The model under review builds one solid part; all positions refer to its coordinate system, in mm. A direction names the side the tool comes from. Give positions to 0.01 mm unless a question says otherwise; leave off trailing zeros. Order: outer loops, then holes, each group sorted by start corner. A loop starts at its lowest first (then second) coordinate and runs counter-clockwise, first axis right, second up. Notation, with made-up numbers: (70, 73) - (125, 73) arc R17 cw to (125, 84) - close; hole circle Ø5 at (69.5, 81). An arc over 180 degrees is marked (long way). Use CSV: the item, a comma, the result in double quotes.
```python
from build123d import *

# Parameters (mm, degrees)
MASTER_SKETCH_R       = 52.451
MASTER_SKETCH_R_2     = 9.525
MASTER_SKETCH_R_3     = 27.4955
MASTER_SKETCH_R_4     = 6.5
BOSS_EXTRUDE2_DEPTH   = 4.7625
F_5_0MM_DOWEL_HOLE1_D = 5
CIRPATTERN4_COUNT     = 4
M6_CLEARANCE_HOLE4_D  = 6.6
M8_CLEARANCE_HOLE1_D  = 9
CIRPATTERN3_COUNT     = 9
CUT_EXTRUDE2_DEPTH    = 281.006585399
CUT_EXTRUDE3_DEPTH    = 281.006585399
FILLET1_R             = 2.54


with BuildPart() as part:
    # Master Sketch → Boss-Extrude2 (new, symmetric)
    # profile 1 of 5: a face of its own
    with BuildSketch(Plane(origin=(0, 0, 0), x_dir=(1, 0, 0), z_dir=(0, 1, 0))):
        with BuildLine():
            ThreePointArc((-8.636, 127), (-36.396097826, 84.787887478), (-86.152093601, 93.552952189))
            Line((-86.152093601, 93.552952189), (-6.534964144, 18.470363023))
            ThreePointArc((-6.534964144, 18.470363023), (-3.773598517, 34.145603423), (9.525, 25.4))
            ThreePointArc((9.525, 25.4), (8.799952547, 21.754940307), (6.735192091, 18.664807909))
            Line((6.735192091, 18.664807909), (23.243231805, 35.172847623))
            ThreePointArc((23.243231805, 35.172847623), (46.587798651, 48.47044475), (73.449951392, 48.001786374))
            Line((73.449951392, 48.001786374), (207.780426054, 8.637567885))
            ThreePointArc((207.780426054, 8.637567885), (203.365353978, 24.134749361), (219.252182081, 21.439533608))
            Line((219.252182081, 21.439533608), (190.024652545, 91.633132973))
            ThreePointArc((190.024652545, 91.633132973), (188.9083984, 102.577169262), (194.028954622, 112.313588397))
            Line((194.028954622, 112.313588397), (211.918529766, 130.503579499))
            ThreePointArc((211.918529766, 130.503579499), (196.325302338, 133.542806943), (205.218502749, 146.70702479))
            Line((205.218502749, 146.70702479), (174.268477279, 147.002761769))
            ThreePointArc((174.268477279, 147.002761769), (167.967389572, 148.13899706), (162.39865644, 151.298735696))
            ThreePointArc((162.39865644, 151.298735696), (144.003054669, 161.678519087), (123.19, 165.2778))
            Line((123.19, 165.2778), (-50.637408401, 172.802043535))
            ThreePointArc((-50.637408401, 172.802043535), (-20.726046555, 158.072276629), (-8.636, 127))
        make_face()
        with Locations(Location((123.19, 103.3018, 0), (0, 0, 90))):
            Circle(MASTER_SKETCH_R, mode=Mode.SUBTRACT)
    # profile 2 of 5: a face of its own
    with BuildSketch(Plane(origin=(0, 0, 0), x_dir=(1, 0, 0), z_dir=(0, 1, 0))):
        with Locations((210.458993886, 17.778185992)):
            Circle(MASTER_SKETCH_R_2)
    # profile 3 of 5: a face of its own
    with BuildSketch(Plane(origin=(0, 0, 0), x_dir=(1, 0, 0), z_dir=(0, 1, 0))):
        with Locations((0, 25.4)):
            Circle(MASTER_SKETCH_R_2)
    # profile 4 of 5: a face of its own
    with BuildSketch(Plane(origin=(0, 0, 0), x_dir=(1, 0, 0), z_dir=(0, 1, 0))):
        with Locations((205.12749261, 137.182459595)):
            Circle(MASTER_SKETCH_R_2)
    # profile 5 of 5: a face of its own
    with BuildSketch(Plane(origin=(0, 0, 0), x_dir=(1, 0, 0), z_dir=(0, 1, 0))):
        with BuildLine():
            ThreePointArc((-54.61, 172.974), (-97.337644752, 143.969297274), (-86.152093601, 93.552952189))
            ThreePointArc((-86.152093601, 93.552952189), (-36.396097826, 84.787887478), (-8.636, 127))
            ThreePointArc((-8.636, 127), (-20.726046555, 158.072276629), (-50.637408401, 172.802043535))
            Line((-50.637408401, 172.802043535), (-54.61, 172.974))
        make_face()
        with Locations(Location((-54.61, 127, 0), (0, 0, 90))):
            Circle(MASTER_SKETCH_R_3, mode=Mode.SUBTRACT)
        with Locations(Location((-67.94878559, 163.648012211, 0), (0, 0, 90))):
            Circle(MASTER_SKETCH_R_4, mode=Mode.SUBTRACT)
        with Locations(Location((-41.27121441, 163.648012211, 0), (0, 0, 90))):
            Circle(MASTER_SKETCH_R_4, mode=Mode.SUBTRACT)
    extrude(amount=BOSS_EXTRUDE2_DEPTH, both=True)

    # Ø5.0mm Dowel Hole1 (through all)
    with Locations(Plane(origin=(0, 4.7625, 0), x_dir=(1, 0, 0), z_dir=(0, 1, 0))):
        with Locations((123.19, 160.4518)):
            f_5_0mm_dowel_hole1 = Hole(F_5_0MM_DOWEL_HOLE1_D / 2)

    # CirPattern4: Ø5.0mm Dowel Hole1 ×4 about axis
    cirpattern4_axis = Axis((123.19, 0, -103.3018), (0, 1, 0))
    for i in range(1, CIRPATTERN4_COUNT):
        add(f_5_0mm_dowel_hole1.rotate(cirpattern4_axis, i * 360 / CIRPATTERN4_COUNT), mode=Mode.SUBTRACT)

    # M6 Clearance Hole4 (through all)
    with Locations(Plane(origin=(0, 4.7625, 0), x_dir=(1, 0, 0), z_dir=(0, 1, 0))):
        with Locations((205.12749261, 137.182459595), (210.458993886, 17.778185992), (0, 25.4)):
            Hole(M6_CLEARANCE_HOLE4_D / 2)

    # M8 Clearance Hole1 (through all)
    with Locations(Plane(origin=(0, 4.7625, 0), x_dir=(1, 0, 0), z_dir=(0, 1, 0))):
        with Locations((-54.61, 166)):
            m8_clearance_hole1 = Hole(M8_CLEARANCE_HOLE1_D / 2)

    # CirPattern3: M8 Clearance Hole1 ×9 about axis
    cirpattern3_axis = Axis((-54.61, 0, -127), (0, 1, 0))
    for i in range(1, CIRPATTERN3_COUNT):
        add(m8_clearance_hole1.rotate(cirpattern3_axis, i * 360 / CIRPATTERN3_COUNT), mode=Mode.SUBTRACT)

    # Topology 3 → Cut-Extrude2 (cut, through all)
    with BuildSketch(Plane(origin=(0, 4.7625, 0), x_dir=(1, 0, 0), z_dir=(0, 1, 0))):
        with BuildLine():
            ThreePointArc((17.44176984, 42.84176984), (-0.146601343, 35.405008389), (-17.945313453, 42.323250142))
            Line((-17.945313453, 42.323250142), (-33.032755262, 56.551396808))
            ThreePointArc((-33.032755262, 56.551396808), (-37.018106584, 65.604842248), (-33.299725858, 74.771168898))
            Line((-33.299725858, 74.771168898), (-25.157987823, 82.912906934))
            ThreePointArc((-25.157987823, 82.912906934), (-16.98904431, 89.126755018), (-7.457826773, 92.934567826))
            Line((-7.457826773, 92.934567826), (46.455825782, 106.412980965))
            ThreePointArc((46.455825782, 106.412980965), (54.31445648, 104.914466858), (58.258837609, 97.954188236))
            ThreePointArc((58.258837609, 97.954188236), (60.562629767, 85.344481192), (65.290751922, 73.429908983))
            ThreePointArc((65.290751922, 73.429908983), (65.041767103, 64.243340795), (57.144809578, 59.543012047))
            ThreePointArc((57.144809578, 59.543012047), (35.149119712, 54.590587492), (16.508039714, 41.908039714))
            Line((16.508039714, 41.908039714), (17.44176984, 42.84176984))
        make_face()
        with BuildLine():
            ThreePointArc((70.803785714, 158.011455607), (76.396746832, 154.095181656), (75.205983312, 147.372050096))
            ThreePointArc((75.205983312, 147.372050096), (73.43400978, 145.361213194), (71.746239826, 143.279197866))
            ThreePointArc((71.746239826, 143.279197866), (68.65233257, 140.432136587), (64.798418838, 138.751253195))
            Line((64.798418838, 138.751253195), (7.651359628, 124.464488392))
            ThreePointArc((7.651359628, 124.464488392), (-0.093621954, 125.882803807), (-4.12477238, 132.646396384))
            ThreePointArc((-4.12477238, 132.646396384), (-5.583091379, 140.304218545), (-8.195896476, 147.648752845))
            ThreePointArc((-8.195896476, 147.648752845), (-7.366745421, 156.880779005), (0.918658655, 161.03648325))
            Line((0.918658655, 161.03648325), (70.803785714, 158.011455607))
        make_face()
        with BuildLine():
            ThreePointArc((153.7341925, 45.75438385), (167.575229688, 55.608989362), (178.397536188, 68.70728094))
            ThreePointArc((178.397536188, 68.70728094), (184.302356988, 71.663840908), (189.640513132, 67.776393867))
            Line((189.640513132, 67.776393867), (204.070964881, 33.119843524))
            ThreePointArc((204.070964881, 33.119843524), (202.654674642, 24.77158437), (194.511168192, 22.451538756))
            Line((194.511168192, 22.451538756), (154.925497425, 34.05172849))
            ThreePointArc((154.925497425, 34.05172849), (150.393857669, 39.502381203), (153.7341925, 45.75438385))
        make_face()
        with BuildLine():
            Line((190.422266455, 122.2302916), (194.644093936, 126.523015363))
            ThreePointArc((194.644093936, 126.523015363), (195.984862679, 133.402037195), (190.177409258, 137.325312223))
            Line((190.177409258, 137.325312223), (184.156778477, 137.382841196))
            ThreePointArc((184.156778477, 137.382841196), (181.428820013, 135.882340302), (181.294822723, 132.771825065))
            ThreePointArc((181.294822723, 132.771825065), (183.396981456, 128.197024139), (185.139600999, 123.473555924))
            ThreePointArc((185.139600999, 123.473555924), (187.431229964, 121.366022532), (190.422266455, 122.2302916))
        make_face()
    extrude(amount=-CUT_EXTRUDE2_DEPTH, mode=Mode.SUBTRACT)

    # Sketch29 → Cut-Extrude3 (cut, through all)
    with BuildSketch(Plane.XZ.offset(4.7625)):
        with BuildLine():
            Line((-72.305646266, -158.824345033), (-79.713448931, -165.515263569))
            ThreePointArc((-79.713448931, -165.515263569), (-70.954498766, -169.970525201), (-61.44878559, -172.462508594))
            Line((-61.44878559, -172.462508594), (-61.44878559, -163.648012211))
            ThreePointArc((-61.44878559, -163.648012211), (-70.587952655, -169.588112984), (-72.305646266, -158.824345033))
        make_face()
        with BuildLine():
            Line((-47.77121441, -163.648012211), (-47.77121441, -172.677978281))
            Line((-47.77121441, -172.677978281), (-34.77121441, -172.115263995))
            Line((-34.77121441, -172.115263995), (-34.77121441, -163.648012211))
            ThreePointArc((-34.77121441, -163.648012211), (-41.27121441, -170.148012211), (-47.77121441, -163.648012211))
        make_face()
    extrude(amount=-CUT_EXTRUDE3_DEPTH, mode=Mode.SUBTRACT)

    # Fillet1
    fillet1_edges = [part.edges().sort_by_distance(p)[0] for p in [
        (-61.44878559, 0, -172.462508594),
        (-79.713448931, 0, -165.515263569),
        (-34.77121441, 0, -172.115263995),
        (-47.77121441, 0, -172.677978281),
    ]]
    fillet(fillet1_edges, radius=FILLET1_R)


solid = part.part
```
Item 1: Take a section at B-B, the plane x = 134. Give the boundary of the cut face in (y, z).
Results list:
outline,"(-4.76, -164.33) - (4.76, -164.33) - (4.76, -154.63) - (-4.76, -154.63) - close; (-4.76, -51.98) - (4.76, -51.98) - (4.76, -30.26) - (-4.76, -30.26) - close"
Item 2: Take a section at C-C, the plane y = 2. State how many separate pieces and enclosed holes the cut face has, and give its area (3 significant figures).
Results list:
separate pieces,"1"
enclosed holes,"22"
area,"16,500 mm2"
Item 3: Clearance check with flat-ended pins moving along their axes: pin 1 (2 mm diameter, centred on x = 5.5, y = 3, fed in from +Z) (3 decimals); pin 2 (5.5 mm diameter, centred on x = 210.46, z = -17.78, fed in from -Y); pin 3 (1.5 mm diameter, centred on x = 162.5, y = -3, fed in from -Z); pin 4 (5 mm diameter, centred on y = 1.5, z = -82.5, fed in from +X). State where each tip first meets the part, or that it passes through.
Results list:
pin 1,"stops at z = -17.005"
pin 2,"passes through"
pin 3,"stops at z = -151.82"
pin 4,"stops at x = 194.87"
Item 4: Wall thickness on L1, parallel to Z at x = 191, y = 1.5; L2, parallel to X at y = -4.5, z = -84.5; L3, parallel to X at y = -1.75, z = -64: over which ranges is each line inside the solid? List them lowest first.
Results list:
L1,"z = -146.84 to -137.26, -122.82 to -108.28, -89.29 to -64.51, -23.48 to -13.55"
L2,"x = -76.55 to -23.47, 60.81 to 74.22, 172.16 to 192.99"
L3,"x = -54.81 to -36.89, 64.89 to 88.46, 157.92 to 175.15, 191.21 to 201.53"
Item 5: Take a section at A-A, the plane z = -25.4. Give the boundary of the cut face in (x, y), and give its area (3 significant figures).
Results list:
outline,"(-13.88, -4.76) - (-3.3, -4.76) - (-3.3, 4.76) - (-13.88, 4.76) - close; (3.3, -4.76) - (13.47, -4.76) - (13.47, 4.76) - (3.3, 4.76) - close; (150.58, -4.76) - (184.45, -4.76) - (184.45, 4.76) - (150.58, 4.76) - close; (203.16, -4.76) - (217.6, -4.76) - (217.6, 4.76) - (203.16, 4.76) - close"
area,"658 mm2"
Item 6: Mouldability with a two-part tool opening along X and no side actions: class faces 3 (the face through (-100.44, 0.07, -130.64)), 4 (the face through (144.28, -0.07, -161.58)), 5 (the face through (-34.771, 0, -167)) as pulls with the +X half, pulls with the -X half, needs draft (parallel to the pull), parting line crosses it, or undercut.
Results list:
face 3,"pulls with the -X half"
face 4,"pulls with the +X half"
face 5,"undercut"
Item 7: Tool access review of faces 1 (the face through (-25.383, 0.067, -49.338)), 2 (the face through (188.88, -0.07, -102.42)): name each direction out of +Z, -Z, +X, -X, +Y, -Y from which nothing blocks a thin tool from reaching the whole face with its end or side.
Results list:
face 1,"+Y, -Y"
face 2,"+X, +Y, -Y"
